Could you check a few things on this model? Use its own coordinates, in mm. A direction names the side the tool comes from. Give positions to 0.01 mm unless a question says otherwise; leave off trailing zeros. Order: outer loops, then holes, each group sorted by start corner. A loop starts at its lowest first (then second) coordinate and runs counter-clockwise, first axis right, second up.
(1) Imagine slicing it at C-C, the plane y = 13. Write out the boundary of the cut face in (x, z), then the cut area to 3 significant figures.
(2) If we mould it in two halves opening along Y, with no side actions, what happens to faces 5 (the flat face through (27, 1, 22)), 6 (the flat face through (32, 10, 19)), 7 (the cylindrical face through (-25.494, 0.533, 29.297)), 8 (the cylindrical face through (30.92, 5.42, 24.01))? For each: released by +Y, released by -Y, zero draft, split by the parting line, or undercut.
(3) Will these pins go through, and if not, where does the flat tip stop? pin 1 (5 mm diameter, centred on x = -52.5, y = -1, fed in from +Z); pin 2 (3.5 mm diameter, centred on x = -102.5, z = 19, fed in from +Y); pin 3 (4.5 mm diameter, centred on x = 30, y = 4, fed in from -Z).
(4) Imagine slicing it at D-D, the plane x = 6.5. Write out the boundary of the cut face in (y, z), then the cut area to 3 significant figures.
(5) Imagine slicing it at A-A, the plane z = 17.5. Write out the boundary of the cut face in (x, y) (1 decimal).
(6) On a 3-axis mill with a long thin cutter (end or side, diameter ignored), from which of +Z, -Z, +X, -X, +Y, -Y can I reach the whole of each face in a straight line? I mean faces 1 (the cylindrical face through (-70, 0, 18)), 2 (the flat face through (34, -10, 19)), 3 (the flat face through (-115, 6, 11)), 4 (the flat face through (-116, 9, 22)). Say none if no direction works.
(7) If I drill on probe 1 along Y at (x, z) = (0, 33); probe 2 along X at (y, z) = (-5, 19) (3 decimals); probe 3 along Z at (x, y) = (-118.5, 10.5), over which ranges is the centre line in solid material (lowest first)?
(8) Imagine slicing it at B-B, the plane y = 4. Write out the boundary of the cut face in (x, z).
from build123d import *

# Parameters (mm, degrees)
BOSS_EXTRUDE1_DEPTH             = 44
BOSS_EXTRUDE2_DEPTH             = 15
BOSS_EXTRUDE3_DEPTH             = 22
BOSS_EXTRUDE4_START             = 10
BOSS_EXTRUDE4_DEPTH             = 24
FILLET1_RADIUS                  = 12
FILLET1_LENGTH                  = 9
FILLET2_RADIUS                  = 12
FILLET2_LENGTH                  = 9
F_6_0MM_DOWEL_HOLE1_D           = 6
F_6_0MM_DOWEL_HOLE1_CSINK_D     = 6.05
F_6_0MM_DOWEL_HOLE1_CSINK_ANGLE = 90


with BuildPart() as part:
    # Sketch1 → Boss-Extrude1 (new body)
    with BuildSketch(Plane.XY):
        with BuildLine():
            Line((0, 25.5), (-2.000483947, 25.421409559))
            ThreePointArc((-2.000483947, 25.421409559), (-25.5, 0), (-2.000483947, -25.421409559))
            Line((-2.000483947, -25.421409559), (0, -25.5))
            ThreePointArc((0, -25.5), (14.05791592, -21.274985311), (23.457408211, -10))
            ThreePointArc((23.457408211, -10), (24.879246203, -5.592236438), (25.480384612, -1))
            Line((25.480384612, -1), (15.835957699, -1))
            ThreePointArc((15.835957699, -1), (-15.8675, 0), (15.835957699, 1))
            Line((15.835957699, 1), (25.480384612, 1))
            ThreePointArc((25.480384612, 1), (24.879246203, 5.592236438), (23.457408211, 10))
            ThreePointArc((23.457408211, 10), (14.05791592, 21.274985311), (0, 25.5))
        make_face()
    extrude(amount=BOSS_EXTRUDE1_DEPTH)

    # Sketch1<3> → Boss-Extrude2 (add)
    with BuildSketch(Plane.XY):
        with BuildLine():
            Line((-2.000483947, 25.421409559), (-140, 20))
            Line((-140, 20), (-90, 20))
            ThreePointArc((-90, 20), (-70, 0), (-90, -20))
            Line((-90, -20), (-140, -20))
            Line((-140, -20), (-2.000483947, -25.421409559))
            ThreePointArc((-2.000483947, -25.421409559), (-25.5, 0), (-2.000483947, 25.421409559))
        make_face()
    extrude(amount=BOSS_EXTRUDE2_DEPTH)

    # Sketch1<4> → Boss-Extrude3 (add)
    with BuildSketch(Plane.XY):
        with BuildLine():
            Line((-140, -20), (-90, -20))
            ThreePointArc((-90, -20), (-70, 0), (-90, 20))
            Line((-90, 20), (-140, 20))
            ThreePointArc((-140, 20), (-160, 0), (-140, -20))
        make_face()
        with BuildLine():
            ThreePointArc((-140, 6), (-146, 0), (-140, -6))
            Line((-140, -6), (-90, -6))
            ThreePointArc((-90, -6), (-84, 0), (-90, 6))
            Line((-90, 6), (-140, 6))
        make_face(mode=Mode.SUBTRACT)
    extrude(amount=BOSS_EXTRUDE3_DEPTH)

    # Sketch1<5> → Boss-Extrude4 (add)
    with BuildSketch(Plane.XY.offset(BOSS_EXTRUDE4_START)):
        with BuildLine():
            Line((44, 10), (23.457408211, 10))
            ThreePointArc((23.457408211, 10), (24.879246203, 5.592236438), (25.480384612, 1))
            Line((25.480384612, 1), (44, 1))
            Line((44, 1), (44, 10))
        make_face()
        with BuildLine():
            ThreePointArc((25.480384612, -1), (24.879246203, -5.592236438), (23.457408211, -10))
            Line((23.457408211, -10), (44, -10))
            Line((44, -10), (44, -1))
            Line((44, -1), (25.480384612, -1))
        make_face()
    extrude(amount=BOSS_EXTRUDE4_DEPTH)

    # Fillet1: full round fillet: the end face becomes a half cylinder, R = half its width
    fillet1_face = Plane((44, 5.5, 22), x_dir=(0, 1, 0), z_dir=(1, 0, 0))  # on the end face: x along it, z out of the body
    fillet1_slab = fillet1_face.offset(-FILLET1_RADIUS / 2) * Box(FILLET1_LENGTH, 2 * FILLET1_RADIUS, FILLET1_RADIUS, mode=Mode.PRIVATE)  # the body's end, R deep
    fillet1_round = Plane((32, 5.5, 22), x_dir=(1, 0, 0), z_dir=(0, 1, 0)) * Cylinder(FILLET1_RADIUS, FILLET1_LENGTH, mode=Mode.PRIVATE)  # its axis R under the face
    add(fillet1_slab - fillet1_round, mode=Mode.SUBTRACT)

    # Fillet2: full round fillet: the end face becomes a half cylinder, R = half its width
    fillet2_face = Plane((44, -5.5, 22), x_dir=(0, -1, 0), z_dir=(1, 0, 0))  # on the end face: x along it, z out of the body
    fillet2_slab = fillet2_face.offset(-FILLET2_RADIUS / 2) * Box(FILLET2_LENGTH, 2 * FILLET2_RADIUS, FILLET2_RADIUS, mode=Mode.PRIVATE)  # the body's end, R deep
    fillet2_round = Plane((32, -5.5, 22), x_dir=(1, 0, 0), z_dir=(0, -1, 0)) * Cylinder(FILLET2_RADIUS, FILLET2_LENGTH, mode=Mode.PRIVATE)  # its axis R under the face
    add(fillet2_slab - fillet2_round, mode=Mode.SUBTRACT)

    # Ø6.0mm Dowel Hole1 (through all)
    with Locations(Plane(origin=(0, 10, 0), x_dir=(1, 0, 0), z_dir=(0, 1, 0))):
        with Locations((33.693220204, -22.863908444)):
            CounterSinkHole(F_6_0MM_DOWEL_HOLE1_D / 2, F_6_0MM_DOWEL_HOLE1_CSINK_D / 2, counter_sink_angle=F_6_0MM_DOWEL_HOLE1_CSINK_ANGLE)


solid = part.part
Answer block:
1. outline: (-155.2, 0) - (-9.1, 0) - (-9.1, 44) - (-21.94, 44) - (-21.94, 15) - (-74.8, 15) - (-74.8, 22) - (-155.2, 22) - close; (9.1, 0) - (21.94, 0) - (21.94, 44) - (9.1, 44) - close
1. area: 3,690 mm2
2. face 5: undercut
2. face 6: released by +Y
2. face 7: split by the parting line
2. face 8: zero draft
3. pin 1: stops at z = 15
3. pin 2: stops at y = 20
3. pin 3: stops at z = 10
4. outline: (-24.66, 0) - (-14.48, 0) - (-14.48, 44) - (-24.66, 44) - close; (14.48, 0) - (24.66, 0) - (24.66, 44) - (14.48, 44) - close
4. area: 896 mm2
5. outline: (-140, -20) - (-90, -20) arc R20 ccw to (-90, 20) - (-140, 20) arc R20 ccw to start; (-2, -25.4) - (0, -25.5) arc R25.5 ccw to (23.5, -10) - (43.1, -10) - (43.1, -1) - (15.8, -1) arc R15.9 cw (long way) to (15.8, 1) - (43.1, 1) - (43.1, 10) - (23.5, 10) arc R25.5 ccw to (0, 25.5) - (-2, 25.4) arc R25.5 ccw to start; hole (-140, -6) - (-90, -6) arc R6 ccw to (-90, 6) - (-140, 6) arc R6 ccw to start
6. face 1: +Z
6. face 2: +Z, -Z, +X, -Y
6. face 3: +Z, -Z
6. face 4: +Z, -X, +Y, -Y
7. probe 1: y = -25.5 to -15.87, 15.87 to 25.5
7. probe 2: x = -159.365 to -143.317, -86.683 to -70.635, -25.005 to -15.059, 15.059 to 43.619
7. probe 3: z = 0 to 22
8. outline: (-159.6, 0) - (-144.47, 0) - (-144.47, 22) - (-159.6, 22) - close; (-85.53, 0) - (-15.36, 0) - (-15.36, 44) - (-25.18, 44) - (-25.18, 15) - (-70.4, 15) - (-70.4, 22) - (-85.53, 22) - close; (15.36, 0) - (25.18, 0) - (25.18, 10) - (32, 10) arc R12 ccw to (32, 34) - (25.18, 34) - (25.18, 44) - (15.36, 44) - close; hole circle Ø6 at (33.69, 22.86)
